Check sheet for the modelled part. Datum: model origin and axes. Units: mm. Face numbers are marked on the shaded views. A direction names the side the tool comes from. Coordinates: 2 decimals unless noted, no trailing zeros. Loops run counter-clockwise (first coordinate to the right, second up) from the corner with the lowest first, then second, coordinate; pieces in that order, holes last.
```python
from build123d import *

# Parameters (mm, degrees)
CUT_EXTRUDE_4_DEPTH      = 9
PATTERN_CIRCULAR_1_COUNT = 6


with BuildPart() as part:
    # 草图1 → 旋转1 (revolve)
    with BuildSketch(Plane.XY):
        Polygon((-16, 52.038271605), (-27.803703704, 52.038271605), (-35, 44.841975309), (-35, 2.038271605), (-30, 2.038271605), (-30, 42.770907497), (-25.732635892, 47.038271605), (-18.250236606, 47.038271605), align=None)
    revolve(axis=Axis((0, 88.586419753, 0), (0, -1, 0)))

    # 草图2 → 切除-拉伸4 (cut)
    with BuildSketch(Plane.XY.offset(40)):
        with BuildLine():
            Line((-4, 52.038271605), (-4, 30.038271605))
            ThreePointArc((-4, 30.038271605), (0, 26.038271605), (4, 30.038271605))
            Line((4, 30.038271605), (4, 52.038271605))
            Line((4, 52.038271605), (-4, 52.038271605))
        make_face()
    cut_extrude_4 = extrude(amount=-CUT_EXTRUDE_4_DEPTH, mode=Mode.SUBTRACT)

    # 阵列(圆周)1: 切除-拉伸4 ×6 about axis
    pattern_circular_1_axis = Axis((0, 0, 0), (0, 1, 0))
    for i in range(1, PATTERN_CIRCULAR_1_COUNT):
        add(cut_extrude_4.rotate(pattern_circular_1_axis, i * 360 / PATTERN_CIRCULAR_1_COUNT), mode=Mode.SUBTRACT)


solid = part.part
```
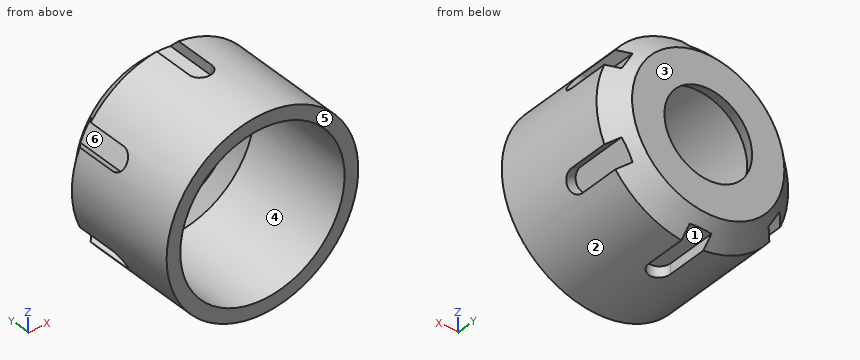
1) Depth check by flat-ended pin: pin 1 (3 mm diameter, centred on y = 38.5, z = -32.5, fed in from +X); pin 2 (5 mm diameter, centred on x = 8, y = 40.5, fed in from +Z); pin 3 (1 mm diameter, centred on x = 14, y = 34.5, fed in from -Z); pin 4 (10 mm diameter, centred on x = 0, z = -27.5, fed in from -Y). Enter the tip coordinate at first touch or a pass-through.
Answer sheet:
pin 1: stops at x = 16.25
pin 2: stops at z = 34.57
pin 3: stops at z = -32.29
pin 4: stops at y = 2.04
2) Section check C-C on y = 32. Enter the section's corners in (x, z), plus the area to 3 significant figures.
Answer sheet:
outline: (-32.11, -13.92) - (-28.85, -12.04) - (-24.85, -18.96) - (-28.11, -20.85) arc R35 ccw to (-4, -34.77) - (-4, -31) - (4, -31) - (4, -34.77) arc R35 ccw to (28.11, -20.85) - (24.85, -18.96) - (28.85, -12.04) - (32.11, -13.92) arc R35 ccw to (32.11, 13.92) - (28.85, 12.04) - (24.85, 18.96) - (28.11, 20.85) arc R35 ccw to (4, 34.77) - (4, 31) - (-4, 31) - (-4, 34.77) arc R35 ccw to (-28.11, 20.85) - (-24.85, 18.96) - (-28.85, 12.04) - (-32.11, 13.92) arc R35 ccw to start; hole circle Ø60 at (0, 0)
area: 833 mm2
3) Set-up check for the marked faces 4, 5 and 6: record each of +Z, -Z, +X, -X, +Y, -Y from which the full face is reachable in a straight line by a thin tool's end or side.
Answer sheet:
face 4: -Y
face 5: +Z, -Z, +X, -X, -Y
face 6: +Y
4) Section check D-D on y = 25. Enter the section's corners in (x, z).
Answer sheet:
outline: circle Ø70 at (0, 0); hole circle Ø60 at (0, 0)
5) Section check B-B on z = 0. Enter the section's corners in (x, y).
Answer sheet:
outline: (-35, 2.04) - (-30, 2.04) - (-30, 42.77) - (-25.73, 47.04) - (-18.25, 47.04) - (-16, 52.04) - (-27.8, 52.04) - (-35, 44.84) - close; (16, 52.04) - (18.25, 47.04) - (25.73, 47.04) - (30, 42.77) - (30, 2.04) - (35, 2.04) - (35, 44.84) - (27.8, 52.04) - close
6) Scan lines: line 1 (X direction, y = 12, z = 0); line 2 (X direction, y = 32, z = -12.5). Record each from-to range of solid material in increasing order.
Answer sheet:
line 1: x = -35 to -30, 30 to 35
line 2: x = -32.69 to -29.65, -28.58 to -27.27, 27.27 to 28.58, 29.65 to 32.69
7) Section check A-A on x = 0. Enter the section's corners in (y, z), plus the area to 3 significant figures.
Answer sheet:
outline: (2.04, -35) - (26.04, -35) - (26.04, -31) - (48.84, -31) - (52.04, -27.8) - (52.04, -16) - (47.04, -18.25) - (47.04, -25.73) - (42.77, -30) - (2.04, -30) - close; (2.04, 30) - (42.77, 30) - (47.04, 25.73) - (47.04, 18.25) - (52.04, 16) - (52.04, 27.8) - (48.84, 31) - (26.04, 31) - (26.04, 35) - (2.04, 35) - close
area: 429 mm2
8) Mould release check, pull along X, two halves, no side actions. Record for the marked faces 1, 2 and 3: +X half, -X half, draft (parallel to the pull), parting line (faces both ways), or undercut.
Answer sheet:
face 1: undercut
face 2: parting line
face 3: draft
